Can you work these out from the drawing? Everything is in mm from the part's minimum corner. A direction names the side the tool comes from. Give positions to 0.01 mm unless a question says otherwise; leave off trailing zeros. Order: outer loops, then holes, each group sorted by start corner. A loop starts at its lowest first (then second) coordinate and runs counter-clockwise, first axis right, second up. Notation, with made-up numbers: (68, 9.5) - (75, 9.5) arc R17 ccw to (75, 30.5) - close; hole circle Ø4 at (89.5, -11.5). An arc over 180 degrees is marked (long way). One line per question, with ' | ' between items.
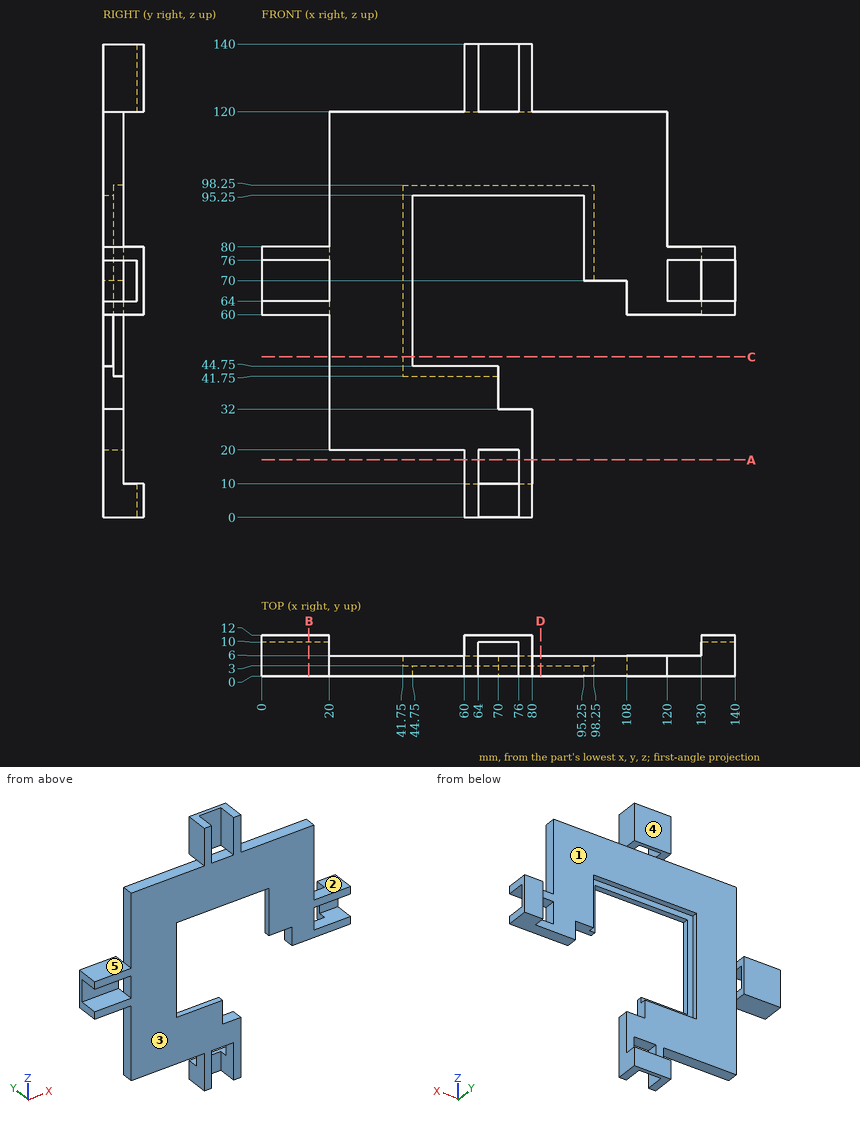
(1) Imagine slicing it at A-A (z = 17). List the corners of the cut face in (x, y) for me, and give its area (3 significant figures).
Answer below:
outline: (60, 0) - (64, 0) - (64, 6) - (60, 6) - close; (76, 0) - (80, 0) - (80, 6) - (76, 6) - close | area: 48.0 mm^2
(2) Will these pins go through, and if not, where does the flat tip stop? pin 1 (3 mm diameter, centred on y = 3, z = 126.5, fed in from +X); pin 2 (5 mm diameter, centred on y = 4.5, z = 39, fed in from +X); pin 3 (6 mm diameter, centred on x = 92, y = 1.5, fed in from -Z); pin 4 (1.8 mm diameter, centred on y = 4.5, z = 63, fed in from -X).
Answer below:
pin 1: x = 80 | pin 2: x = 70 | pin 3: z = 95.25 | pin 4: x = 0
(3) On a 3-axis mill with a long thin cutter (end or side, diameter ignored), from which of +Z, -Z, +X, -X, +Y, -Y can I reach the whole of each face in a straight line? I mean the marked faces 1, 2, 3, 4 and 5. Say none if no direction works.
Answer below:
face 1: +Y | face 2: +Z, +X, +Y, -Y | face 3: +Z, -Z, +X, -X, -Y | face 4: +Z, -Z, +X, -X, +Y | face 5: +Z, -X, +Y, -Y
(4) Imagine slicing it at B-B (x = 14). List the corners of the cut face in (y, z) for me.
Answer below:
outline: (0, 60) - (12, 60) - (12, 80) - (0, 80) - (0, 76) - (10, 76) - (10, 64) - (0, 64) - close
(5) Imagine slicing it at C-C (z = 47.5). List the corners of the cut face in (x, y) for me, and give its area (4 significant figures).
Answer below:
outline: (20, 0) - (44.75, 0) - (44.75, 3) - (41.75, 3) - (41.75, 6) - (20, 6) - close | area: 139.5 mm^2
(6) If I drill on line 1 (Z direction, x = 68, y = 5.5); line 2 (X direction, y = 1, z = 130.5); line 3 (X direction, y = 1.5, z = 93), over which ranges is the centre line in solid material (lowest first)?
Answer below:
line 1: 20 to 41.75, 98.25 to 120 | line 2: 60 to 64, 76 to 80 | line 3: 20 to 44.75, 95.25 to 120
(7) Imagine slicing it at D-D (x = 82.5). List the corners of the cut face in (y, z) for me, and give its area (4 significant figures).
Answer below:
outline: (0, 95.25) - (3, 95.25) - (3, 98.25) - (6, 98.25) - (6, 120) - (0, 120) - close | area: 139.5 mm^2
